Input: dimensioned drawing with shaded views. Units: mm. Origin: part minimum x, y, z. Coordinates: 2 decimals unless noted, no trailing zeros. Order: outer loops, then holes, each group sorted by start corner. A loop starts at its lowest first (then second) coordinate and runs counter-clockwise, first axis right, second up. Notation, with made-up numbers: (79.25, 45.25) - (124.25, 45.25) arc R28 cw to (124.25, 74.25) - close; hole circle Ø9 at (-14, -14.75). An arc over 180 degrees is marked (long way). One line per question, with ' | ' between items. Start each with the question number.
(1) Line query: line 1 along X through (y, z) = (3.75, 71); line 2 along Z through (x, y) = (39.5, 0.75) (3 decimals); line 3 along X through (y, z) = (3, 41). Output: solid intervals per line, ascending.
(2) Section B-B (x = 174). Return the cut outline in (y, z) (3 decimals), then the cut area to 3 significant figures.
(3) Section D-D (x = 109). Return the cut outline in (y, z), then the cut area to 3 significant figures.
(4) Contact query for a flat-ended pin moving along its axis: P1, Ø3, axis at y = 3.5, z = 81.5, coming from the -X side. Output: stop coordinate, or through.
(5) Section C-C (y = 4.5). Count the separate pieces of the cut face and the enclosed holes in it, then the cut area to 3 significant figures.
(6) Section A-A (z = 69.5). Return the cut outline in (x, y), then the cut area to 3 significant figures.
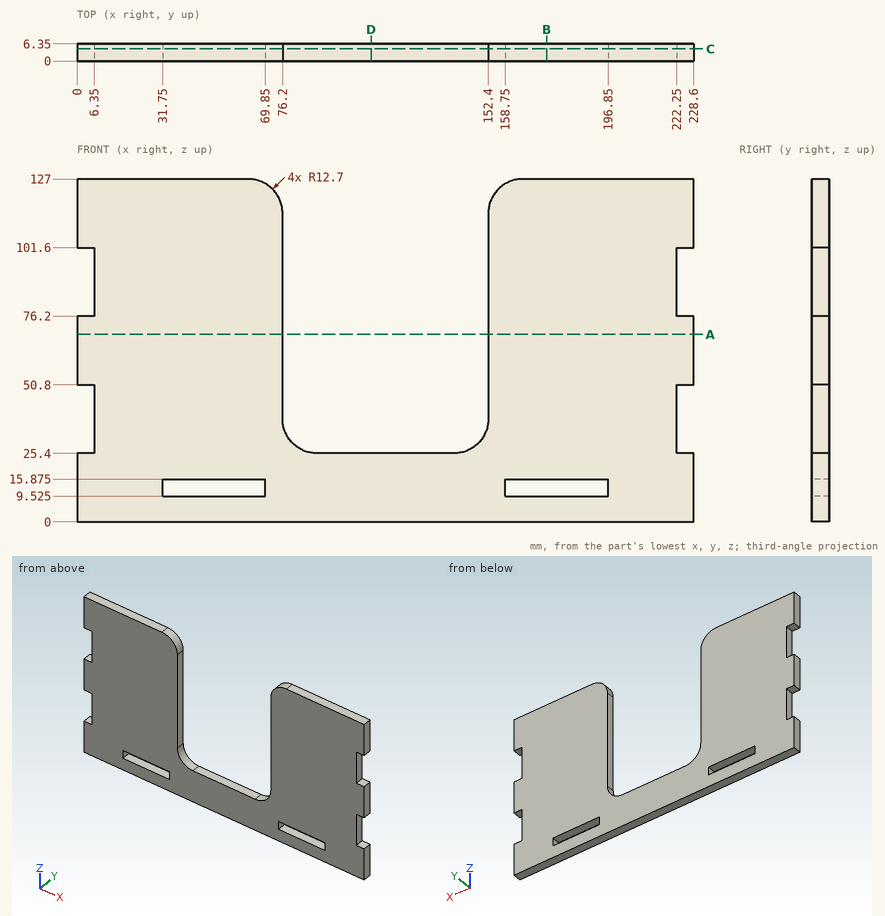
Response values:
1) line 1: x = 0 to 76.2, 152.4 to 228.6 | line 2: z = 0 to 9.525, 15.875 to 127 | line 3: x = 6.35 to 76.2, 152.4 to 222.25
2) outline: (0, 0) - (6.35, 0) - (6.35, 9.525) - (0, 9.525) - close; (0, 15.875) - (6.35, 15.875) - (6.35, 127) - (0, 127) - close | area: 766 mm²
3) outline: (0, 0) - (6.35, 0) - (6.35, 25.4) - (0, 25.4) - close | area: 161 mm²
4) P1: stops at x = 6.35
5) separate pieces: 1 | enclosed holes: 2 | area: 20,200 mm²
6) outline: (0, 0) - (76.2, 0) - (76.2, 6.35) - (0, 6.35) - close; (152.4, 0) - (228.6, 0) - (228.6, 6.35) - (152.4, 6.35) - close | area: 968 mm²
